from build123d import *

# Parameters (mm, degrees)
BOSS_EXTRUDE1_DEPTH = 2
SKETCH2_W           = 30
SKETCH2_H           = 10
CUT_EXTRUDE1_DEPTH  = 364.88597115
FILLET1_R           = 3
SKETCH3_R           = 1.6
CUT_EXTRUDE2_DEPTH  = 364.88597115


with BuildPart() as part:
    # Sketch1 → Boss-Extrude1 (new body)
    with BuildSketch(Plane.XY):
        with BuildLine():
            Line((-43, 260), (43, 260))
            ThreePointArc((43, 260), (50.071067812, 262.928932188), (53, 270))
            Line((53, 270), (53, 350))
            ThreePointArc((53, 350), (50.071067812, 357.071067812), (43, 360))
            Line((43, 360), (-43, 360))
            ThreePointArc((-43, 360), (-50.071067812, 357.071067812), (-53, 350))
            Line((-53, 350), (-53, 270))
            ThreePointArc((-53, 270), (-50.071067812, 262.928932188), (-43, 260))
        make_face()
    extrude(amount=-BOSS_EXTRUDE1_DEPTH)

    # Sketch2 → Cut-Extrude1 (cut, through all)
    with BuildSketch(Plane.XY):
        with Locations((0, 355)):
            Rectangle(SKETCH2_W, SKETCH2_H)
    extrude(amount=-CUT_EXTRUDE1_DEPTH, mode=Mode.SUBTRACT)

    # Fillet1
    fillet1_edges = [part.edges().sort_by_distance(p)[0] for p in [
        (-15, 350, -1),
        (15, 350, -1),
    ]]
    fillet(fillet1_edges, radius=FILLET1_R)

    # Sketch3 → Cut-Extrude2 (cut, through all)
    with BuildSketch(Plane.XY):
        with Locations((47, 354)):
            Circle(SKETCH3_R)
        with Locations((47, 266)):
            Circle(SKETCH3_R)
        with Locations(Location((-47, 266, 0), (0, 0, 180))):
            Circle(SKETCH3_R)
        with Locations(Location((-47, 354, 0), (0, 0, 180))):
            Circle(SKETCH3_R)
    extrude(amount=-CUT_EXTRUDE2_DEPTH, mode=Mode.SUBTRACT)


solid = part.part
Model file for the job. Use its own axes, mm. A direction names the side the tool comes from. Give positions to 0.01 mm unless a question says otherwise; leave off trailing zeros. Write each loop counter-clockwise with the first axis right and the second up, starting at its lowest first coordinate (ties: lowest second). Pieces come first, ordered by that corner, then holes. Notation, with made-up numbers: M -23,31.5 L 7,31.5 A17 cw 7,36.5 Z; hole C -33,85.25 d2. An arc over 180 degrees is marked long. One line per item, written item: value. Start each with the question number.
Q1. Two-plate mould, pull along X, no slides. Class faces 3 (the cylindrical face through (46.792, 355.586, -0.986)), 4 (the cylindrical face through (-50.15, 263.01, -0.99)), 5 (the flat face through (-1, 311, 0)): +X half, -X half, draft (parallel to the pull), parting line (faces both ways), or undercut.
Q2. 3-axis set-ups, long thin cutter, end or side, ignore diameter. For faces 1 (the cylindrical face through (-14.14, 350.9, -1.01)), 2 (the cylindrical face through (46.792, 267.586, -0.986)): which of +Z, -Z, +X, -X, +Y, -Y reach the whole face in a straight line?
Q3. Probe probe 1 along X at (y, z) = (266, -0.9); probe 2 along Y at (x, z) = (47, -1.4); probe 3 along X at (y, z) = (354, -0.85). List the from-to ranges inside material, lowest first. Write a range as [from, to].
Q4. Saw through at D-D, the plane x = 2. Write the cut outline in (y, z), plus the area to 3 significant figures.
Q5. Drop flat-ended pins along their axis: pin 1 Ø3.5 at (x, y) = (-47, 266) entering from -Z; pin 2 Ø1 at (y, z) = (358, -1) entering from -X; pin 3 Ø0.6 at (y, z) = (358, -0.5) entering from +X; pin 4 Ø3 at (x, y) = (-47, 354) entering from -Z. Give the stop position or say it passes through.
Q6. Saw through at C-C, the plane y = 266. Write the cut outline in (x, z), plus the area to 3 significant figures.
Q7. Saw through at B-B, the plane x = -47. Write the cut outline in (y, z), plus the area to 3 significant figures.
Q8. Saw through at A-A, the plane z = -0.35. Write the cut outline in (x, y), plus the area to 3 significant figures.
Output values:
1. face 3: undercut
1. face 4: -X half
1. face 5: draft
2. face 1: +Z, -Z, +Y
2. face 2: +Z, -Z
3. probe 1: x = [-52.17, -48.6], [-45.4, 45.4], [48.6, 52.17]
3. probe 2: y = [260.83, 264.4], [267.6, 352.4], [355.6, 359.17]
3. probe 3: x = [-52.17, -48.6], [-45.4, -15], [15, 45.4], [48.6, 52.17]
4. outline: M 260,-2 L 350,-2 L 350,0 L 260,0 Z
4. area: 180 mm²
5. pin 1: stops at z = -2
5. pin 2: stops at x = -49.61
5. pin 3: stops at x = 49.38
5. pin 4: passes through
6. outline: M -52.17,-2 L -48.6,-2 L -48.6,0 L -52.17,0 Z; M -45.4,-2 L 45.4,-2 L 45.4,0 L -45.4,0 Z; M 48.6,-2 L 52.17,-2 L 52.17,0 L 48.6,0 Z
6. area: 196 mm²
7. outline: M 260.83,-2 L 264.4,-2 L 264.4,0 L 260.83,0 Z; M 267.6,-2 L 352.4,-2 L 352.4,0 L 267.6,0 Z; M 355.6,-2 L 359.17,-2 L 359.17,0 L 355.6,0 Z
7. area: 184 mm²
8. outline: M -53,270 A10 ccw -43,260 L 43,260 A10 ccw 53,270 L 53,350 A10 ccw 43,360 L 15,360 L 15,353 A3 cw 12,350 L -12,350 A3 cw -15,353 L -15,360 L -43,360 A10 ccw -53,350 Z; hole C -47,266 d3.2; hole C -47,354 d3.2; hole C 47,266 d3.2; hole C 47,354 d3.2
8. area: 10,200 mm²
